Could you check a few things on this model? Use its own coordinates, in mm. Face numbers are marked on the shaded views. A direction names the side the tool comes from. Coordinates: 2 decimals unless noted, no trailing zeros. Loops run counter-clockwise (first coordinate to the right, second up) from the corner with the lowest first, then second, coordinate; pieces in that order, holes last. Notation, with made-up numbers: M -12.75,13.5 L 33.25,13.5 A24 ccw 33.25,40.5 Z; hole C 74.25,33.5 d6. An arc over 180 degrees is marked long. Return JSON: item names as keys, results as strings. Group by question number.
from build123d import *

# Parameters (mm, degrees)
F2_R = 5.08
F3_R = 5.08


with BuildPart() as f1:
    # F0 (on Front) → F1 (revolve)
    with BuildSketch(Plane.XZ):
        Polygon((-18.6021607369, -9.4218043774), (-29.5509118587, -9.4218043774), (-29.5509118587, -12.5968043774), (33.9490881413, -12.5968043774), (33.9490881413, -3.0718043774), (-8.9451875538, -3.0718043774), align=None)
    revolve(axis=Axis((2.1990881413, 0, -12.5968043774), (1, 0, 0)))

    # F2
    f2_edges = [f1.edges().sort_by_distance(p)[0] for p in [
        (33.949088, 0, -22.121804),
    ]]
    fillet(f2_edges, radius=F2_R)

    # F3
    f3_edges = [f1.edges().sort_by_distance(p)[0] for p in [
        (-8.945188, 0, -22.121804),
        (-18.602161, 0, -15.771804),
        (-13.773674, 0, -6.246804),
    ]]
    fillet(f3_edges, radius=F3_R)


solid = f1.part
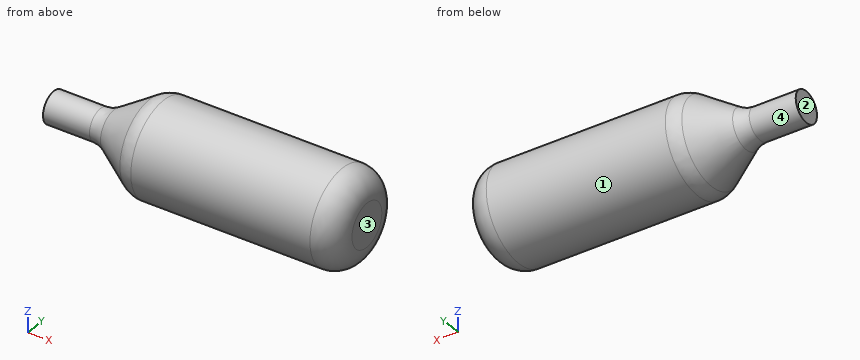
(1) Will these pins go through, and if not, where does the flat tip stop? P1, Ø1, axis at x = -11.5, z = -17.5, coming from the -Y side; P2, Ø5, axis at x = -15.5, y = -1, coming from the -Z side; P3, Ø2, axis at x = 26.5, z = -7, coming from the -Y side.
(2) If I drill on L1, parallel to Y at x = -5.5, z = -5; L2, parallel to X at y = -5.5, z = -15; L3, parallel to Y at x = 12, z = -17, over which ranges is the centre line in solid material (lowest first)? Write a range as [from, to].
(3) For the marked faces 3 and 4, which set-ups out of +Z, -Z, +X, -X, +Y, -Y let a thin tool reach every point of the face, with its end or its side?
(4) Imagine slicing it at B-B, the plane x = 19. Write out the boundary of the cut face in (y, z) (3 decimals), then the cut area to 3 significant figures.
(5) We'd pull the mould along Y, two halves only. Please class the marked faces 1 and 2: +Y half, -Y half, draft (parallel to the pull), parting line (faces both ways), or undercut.
(6) Imagine slicing it at A-A, the plane x = -25.5. Write out the boundary of the cut face in (y, z) (3 decimals).
Checks:
{
 "1": {"P1": "y = -6.68", "P2": "z = -19.41", "P3": "y = -8.34"},
 "2": {"L1": "[-5.75, 5.75]", "L2": "[-14.3, 33.7]", "L3": "[-8.45, 8.45]"},
 "3": {"face 3": "+Z, -Z, +X, +Y, -Y", "face 4": "-X"},
 "4": {"outline": "C 0,-12.597 d19.05", "area": "285 mm²"},
 "5": {"face 1": "parting line", "face 2": "draft"},
 "6": {"outline": "C 0,-12.597 d6.35"}
}
